```python
from build123d import *

# Parameters (mm, degrees)
SKETCH1_W               = 117.516
SKETCH1_H               = 63
SKETCH1_R               = 3.2004
SKETCH1_R_2             = 3
SKETCH1_R_3             = 12
BOSS_EXTRUDE1_DEPTH     = 3.175
CHAMFER1_SIZE           = 4
F_1_4_20_TAPPED_HOLE1_D = 5.1054
F_6_32_TAPPED_HOLE1_D   = 2.7051


with BuildPart() as part:
    # Sketch1 → Boss-Extrude1 (new body)
    with BuildSketch(Plane.XY):
        with Locations((26.758, -14.99999999)):
            Rectangle(SKETCH1_W, SKETCH1_H)
        with Locations((-24, 9.50000001)):
            Circle(SKETCH1_R, mode=Mode.SUBTRACT)
        with Locations((13.423393759, 7.75)):
            Circle(SKETCH1_R_2, mode=Mode.SUBTRACT)
        with Locations((-7, 0)):
            Circle(SKETCH1_R_3, mode=Mode.SUBTRACT)
        with Locations((13.423393759, -7.75)):
            Circle(SKETCH1_R_2, mode=Mode.SUBTRACT)
        with Locations((-24, -40.49999999)):
            Circle(SKETCH1_R, mode=Mode.SUBTRACT)
        with Locations((0, -15.5)):
            Circle(SKETCH1_R_2, mode=Mode.SUBTRACT)
        with Locations((36, -40.49999999)):
            Circle(SKETCH1_R, mode=Mode.SUBTRACT)
        with Locations((36, 9.50000001)):
            Circle(SKETCH1_R, mode=Mode.SUBTRACT)
    extrude(amount=-BOSS_EXTRUDE1_DEPTH)

    # Chamfer1
    chamfer1_edges = [part.edges().sort_by_distance(p)[0] for p in [
        (-32, -46.49999999, -1.5875),
        (-32, 16.50000001, -1.5875),
        (85.516, 16.50000001, -1.5875),
        (85.516, -46.49999999, -1.5875),
    ]]
    chamfer(chamfer1_edges, length=CHAMFER1_SIZE)

    # 1/4-20 Tapped Hole1 (through all)
    with Locations(Plane.XY):
        with Locations((77.516, 9.50000001), (77.516, -40.49999999)):
            Hole(F_1_4_20_TAPPED_HOLE1_D / 2)

    # #6-32 Tapped Hole1 (through all)
    with Locations(Plane.XY):
        with Locations((13.79086472, -15.75179999)):
            Hole(F_6_32_TAPPED_HOLE1_D / 2)


solid = part.part
```
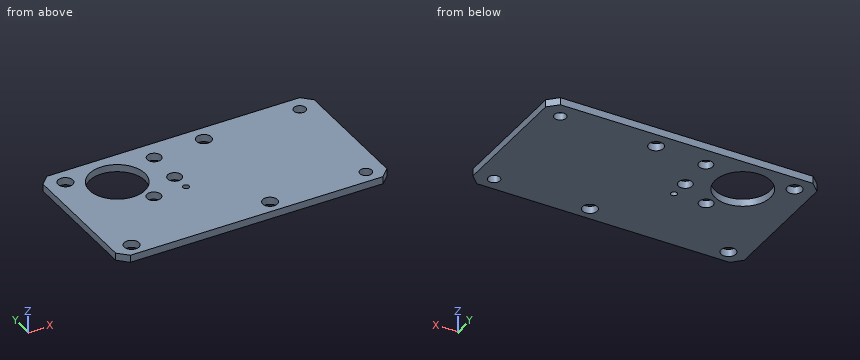
Part model, mm, in its own coordinate system. Round coordinates to 2 decimals unless told otherwise and drop trailing zeros. Loops run counter-clockwise (first coordinate to the right, second up) from the corner with the lowest first, then second, coordinate; pieces in that order, holes last.
1. Slice it at C-C (y = -40.5). Give the cut face in (x, z) (3 decimals), and give its area (3 significant figures).
Solutions:
outline: (-32, -3.175) - (-27.2, -3.175) - (-27.2, 0) - (-32, 0) - close; (-20.8, -3.175) - (32.8, -3.175) - (32.8, 0) - (-20.8, 0) - close; (39.2, -3.175) - (74.963, -3.175) - (74.963, 0) - (39.2, 0) - close; (80.069, -3.175) - (85.516, -3.175) - (85.516, 0) - (80.069, 0) - close
area: 316 mm2
2. Slice it at A-A (x = 36). Give the cut face in (y, z) (3 decimals).
Solutions:
outline: (-46.5, -3.175) - (-43.7, -3.175) - (-43.7, 0) - (-46.5, 0) - close; (-37.3, -3.175) - (6.3, -3.175) - (6.3, 0) - (-37.3, 0) - close; (12.7, -3.175) - (16.5, -3.175) - (16.5, 0) - (12.7, 0) - close
3. Flat gauge pin, fed straight in: pin 1 (6 mm diameter, centred on x = 36, y = -40.5, fed in from -Z). Where does the tip first touch, or does it go through?
Solutions:
pin 1: passes through
4. Slice it at B-B (y = 0). Give the cut face in (x, z) (3 decimals).
Solutions:
outline: (-32, -3.175) - (-19, -3.175) - (-19, 0) - (-32, 0) - close; (5, -3.175) - (85.516, -3.175) - (85.516, 0) - (5, 0) - close
5. Drill centre lines: line 1 along X through (y, z) = (10, -1.75); line 2 along X through (y, z) = (8, -1.85); line 3 along Y through (x, z) = (16, -1.8). Where is each one in solid material? Low to high.
Solutions:
line 1: x = -32 to -27.16, -20.84 to -13.63, -0.37 to 11.44, 15.41 to 32.84, 39.16 to 75.01, 80.02 to 85.52
line 2: x = -32 to -26.83, -21.17 to -15.94, 1.94 to 10.43, 16.41 to 33.17, 38.83 to 75.45, 79.58 to 85.52
line 3: y = -46.5 to -9.29, -6.21 to 6.21, 9.29 to 16.5
6. Slice it at D-D (z = -2.25). Count the separate pieces of the cut face and the enclosed holes in it, and give its area (3 significant figures).
Solutions:
separate pieces: 1
enclosed holes: 11
area: 6,660 mm2
